Answer from the drawing. Dimensions are ordinates in mm from the lowest x, y and z of the part. Round coordinates to 2 decimals unless told otherwise and drop trailing zeros. Loops run counter-clockwise (first coordinate to the right, second up) from the corner with the lowest first, then second, coordinate; pieces in that order, holes last. Notation, with made-up numbers: M 77.5,69.25 L 120.5,69.25 A12 ccw 120.5,78.25 Z; hole C -26.5,48.5 d10. An arc over 180 degrees is marked long. One line per item, written item: value.
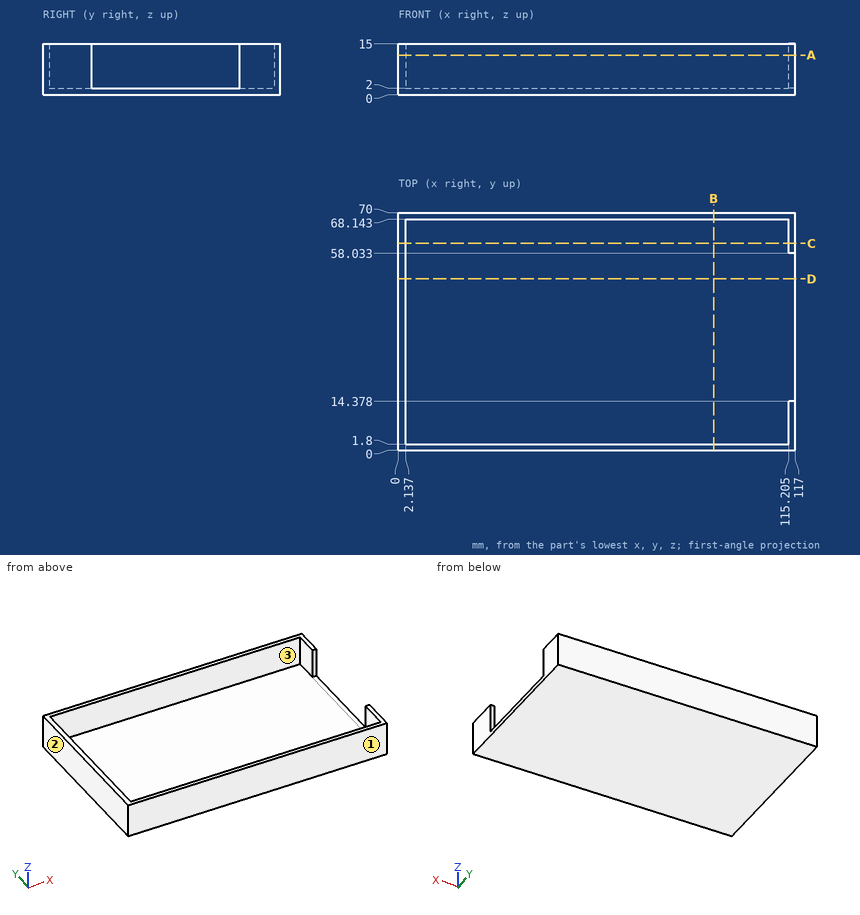
1) Find section D-D (y = 50.5). Give the vertices of the cut face in (x, z), then the cut area to 3 significant figures.
Check values:
outline: M 0,0 L 117,0 L 117,2 L 2.14,2 L 2.14,15 L 0,15 Z
area: 262 mm2
2) Find section B-B (x = 93). Give the vertices of the cut face in (y, z).
Check values:
outline: M 0,0 L 70,0 L 70,15 L 68.14,15 L 68.14,2 L 1.8,2 L 1.8,15 L 0,15 Z
3) Each of these flat-tipped pins is pushed along its axis until it touches: pin 1 (4 mm diameter, centred on x = 80, y = 61.5, fed in from +Z); pin 2 (4 mm diameter, centred on y = 22, z = 10, fed in from +X). Where does it stop, or does it pass through?
Check values:
pin 1: z = 2
pin 2: x = 2.14
4) The mould has two halves that part along Y. Classify the marked faces 1, 2 and 3: +Y half, -Y half, draft (parallel to the pull), parting line (faces both ways), or undercut.
Check values:
face 1: -Y half
face 2: draft
face 3: undercut
5) Find the intervals of material crossed by probe 1 along Y at (x, z) = (100.5, 8); probe 2 along X at (y, z) = (61, 12) (1 decimal); probe 3 along X at (y, z) = (29, 3.75), in increasing order. Write a range as from..to.
Check values:
probe 1: 0..1.8, 68.14..70
probe 2: 0..2.1, 115.2..117
probe 3: 0..2.14
6) Find section C-C (y = 61). Give the vertices of the cut face in (x, z) (1 decimal), then the cut area to 3 significant figures.
Check values:
outline: M 0,0 L 117,0 L 117,15 L 115.2,15 L 115.2,2 L 2.1,2 L 2.1,15 L 0,15 Z
area: 285 mm2
7) Find section A-A (z = 11.75). Give the vertices of the cut face in (x, y) (1 decimal).
Check values:
outline: M 0,0 L 117,0 L 117,14.4 L 115.2,14.4 L 115.2,1.8 L 2.1,1.8 L 2.1,68.1 L 115.2,68.1 L 115.2,58 L 117,58 L 117,70 L 0,70 Z
